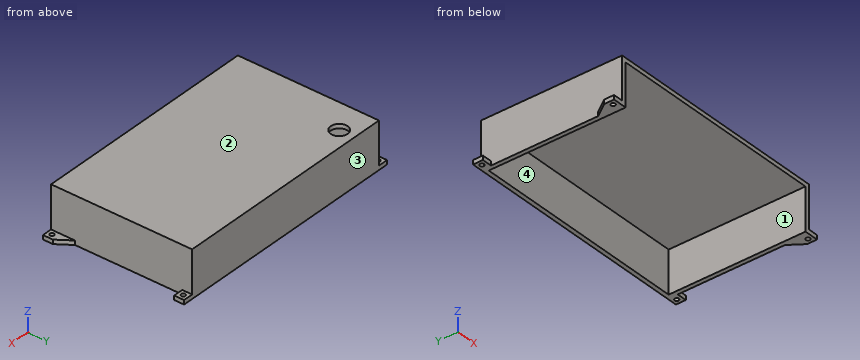
```python
from build123d import *

# Parameters (mm, degrees)
BOSS_EXTRUDE1_DEPTH = 33
SKETCH1_4_R         = 1.5
BOSS_EXTRUDE2_DEPTH = 3
SKETCH3_W           = 156
SKETCH3_H           = 97
CUT_EXTRUDE1_DEPTH  = 30
SKETCH3_4_R         = 6
CUT_EXTRUDE2_DEPTH  = 33


with BuildPart() as part:
    # Sketch1 → Boss-Extrude1 (new body)
    with BuildSketch(Plane.XY):
        Polygon((162, 93), (162, 100), (0, 100), (0, 93), (0, 17), (0, 7), (0, 0), (162, 0), (162, 7), (162, 17), align=None)
    extrude(amount=BOSS_EXTRUDE1_DEPTH)

    # Sketch1_4 → Boss-Extrude2 (add)
    # profile 1 of 6: a face of its own
    with BuildSketch(Plane.XY):
        with BuildLine():
            Line((0, 93), (0, 100))
            Line((0, 100), (-3.5, 100))
            Line((-3.5, 100), (-3.5, 98))
            ThreePointArc((-3.5, 98), (-2.439339828, 97.560660172), (-2, 96.5))
            ThreePointArc((-2, 96.5), (-2.439339828, 95.439339828), (-3.5, 95))
            Line((-3.5, 95), (-3.5, 93))
            Line((-3.5, 93), (0, 93))
        make_face()
    # profile 2 of 6: a face of its own
    with BuildSketch(Plane.XY):
        with BuildLine():
            Line((-3.5, 98), (-3.5, 100))
            Line((-3.5, 100), (-7, 100))
            Line((-7, 100), (-7, 93))
            Line((-7, 93), (-3.5, 93))
            Line((-3.5, 93), (-3.5, 95))
            ThreePointArc((-3.5, 95), (-5, 96.5), (-3.5, 98))
        make_face()
    # profile 3 of 6: a face of its own
    with BuildSketch(Plane.XY):
        Polygon((0, 7), (0, 17), (-7, 7), (-7, 0), (0, 0), align=None)
        with Locations((-3.5, 3.5)):
            Circle(SKETCH1_4_R, mode=Mode.SUBTRACT)
    # profile 4 of 6: a face of its own
    with BuildSketch(Plane.XY):
        Polygon((169, 7), (162, 17), (162, 7), (162, 0), (169, 0), align=None)
        with Locations((165.5, 3.5)):
            Circle(SKETCH1_4_R, mode=Mode.SUBTRACT)
    # profile 5 of 6: a face of its own
    with BuildSketch(Plane.XY):
        with BuildLine():
            Line((169, 100), (165.5, 100))
            Line((165.5, 100), (165.5, 98))
            ThreePointArc((165.5, 98), (166.560660172, 97.560660172), (167, 96.5))
            ThreePointArc((167, 96.5), (166.560660172, 95.439339828), (165.5, 95))
            Line((165.5, 95), (165.5, 93))
            Line((165.5, 93), (169, 93))
            Line((169, 93), (169, 100))
        make_face()
    # profile 6 of 6: a face of its own
    with BuildSketch(Plane.XY):
        with BuildLine():
            Line((165.5, 98), (165.5, 100))
            Line((165.5, 100), (162, 100))
            Line((162, 100), (162, 93))
            Line((162, 93), (165.5, 93))
            Line((165.5, 93), (165.5, 95))
            ThreePointArc((165.5, 95), (164, 96.5), (165.5, 98))
        make_face()
    extrude(amount=BOSS_EXTRUDE2_DEPTH)

    # Sketch3 → Cut-Extrude1 (cut)
    with BuildSketch(Plane(origin=(0, 0, 0), x_dir=(-1, 0, 0), z_dir=(0, 0, -1))):
        with Locations((-81, 48.5)):
            Rectangle(SKETCH3_W, SKETCH3_H)
    extrude(amount=-CUT_EXTRUDE1_DEPTH, mode=Mode.SUBTRACT)

    # Sketch3_4 → Cut-Extrude2 (cut)
    with BuildSketch(Plane(origin=(0, 0, 0), x_dir=(-1, 0, 0), z_dir=(0, 0, -1))):
        with Locations((-21, 89)):
            Circle(SKETCH3_4_R)
    extrude(amount=-CUT_EXTRUDE2_DEPTH, mode=Mode.SUBTRACT)


solid = part.part
```
For this review, take the finished solid that the model builds, in its own axes (mm). Face numbers are marked on the shaded views. A direction names the side the tool comes from. Round coordinates to 2 decimals unless told otherwise and drop trailing zeros. Write each loop counter-clockwise with the first axis right and the second up, starting at its lowest first coordinate (ties: lowest second). Pieces come first, ordered by that corner, then holes. Notation, with made-up numbers: M -31.75,49 L 13.25,49 A19 ccw 13.25,78 Z; hole C 34.25,60.25 d7. An arc over 180 degrees is marked long. One line per item, written item: value. Start each with the question number.
(1) Machinability: for the marked faces 3 and 4, which of the approach directions +Z, -Z, +X, -X, +Y, -Y give a long, thin tool a straight path to every point of the face, cutting with its end or side? Answer none if there is none.
(2) We need section A-A (y = 89). Give the boundary of the cut face in (x, z), and give its area (3 significant figures).
(3) We need section C-C (x = 20.5). Give the boundary of the cut face in (y, z).
(4) We need section D-D (x = 107). Give the boundary of the cut face in (y, z), and give its area (3 significant figures).
(5) We need section B-B (z = 19). Give the boundary of the cut face in (x, y).
(6) Wall thickness on line 1 (X direction, y = 64.5, z = 23); line 2 (Y direction, x = 165.5, z = 2.25); line 3 (X direction, y = 3, z = 1): over which ranges is each line inside the solid? List them lowest first.
(7) Insertion check: pin 1 (5.5 mm diameter, centred on x = 166.5, y = 9, fed in from +Z); pin 2 (2.5 mm diameter, centred on x = -3.5, y = 3.5, fed in from -Z); pin 3 (12 mm diameter, centred on y = 69.5, z = 5.5, fed in from +X); pin 4 (6 mm diameter, centred on x = 41.5, y = 58, fed in from -Z). Each pin has a flat end and moves straight along its axis. Give the tip position at first contact, or say it passes through.
(8) The part is to be moulded in two halves that separate along X. For the marked faces 1 and 2, say which applies: released by +X, released by -X, zero draft, split by the parting line, or undercut.
Result:
1. face 3: +Z, -Z, +X, -X, +Y
1. face 4: -Z, -Y
2. outline: M 0,0 L 3,0 L 3,30 L 15,30 L 15,33 L 0,33 Z; M 27,30 L 159,30 L 159,0 L 162,0 L 162,33 L 27,33 Z
2. area: 630 mm²
3. outline: M 0,30 L 83.02,30 L 83.02,33 L 0,33 Z; M 94.98,30 L 97,30 L 97,0 L 100,0 L 100,33 L 94.98,33 Z
4. outline: M 0,30 L 97,30 L 97,0 L 100,0 L 100,33 L 0,33 Z
4. area: 390 mm²
5. outline: M 0,0 L 3,0 L 3,97 L 159,97 L 159,0 L 162,0 L 162,100 L 0,100 Z
6. line 1: 0 to 3, 159 to 162
6. line 2: 0 to 2, 5 to 12, 93 to 95, 98 to 100
6. line 3: -7 to -4.91, -2.09 to 3, 159 to 164.09, 166.91 to 169
7. pin 1: z = 3
7. pin 2: through
7. pin 3: x = 162
7. pin 4: z = 30
8. face 1: undercut
8. face 2: zero draft
